The figure shows three views and two pictorial views of one solid part (mm, origin at its lowest corner). Answer the questions. A direction names the side the tool comes from. Coordinates: 2 decimals unless noted, no trailing zeros. Write each loop counter-clockwise with the first axis right and the second up, starting at its lowest first coordinate (ties: lowest second). Pieces come first, ordered by that corner, then holes. Notation, with made-up numbers: M 13.25,56 L 22.25,56 A9 ccw 22.25,63 Z; hole C 81,56 d6. An arc over 180 degrees is marked long. Use a Markdown table: item, result. Add a question column.
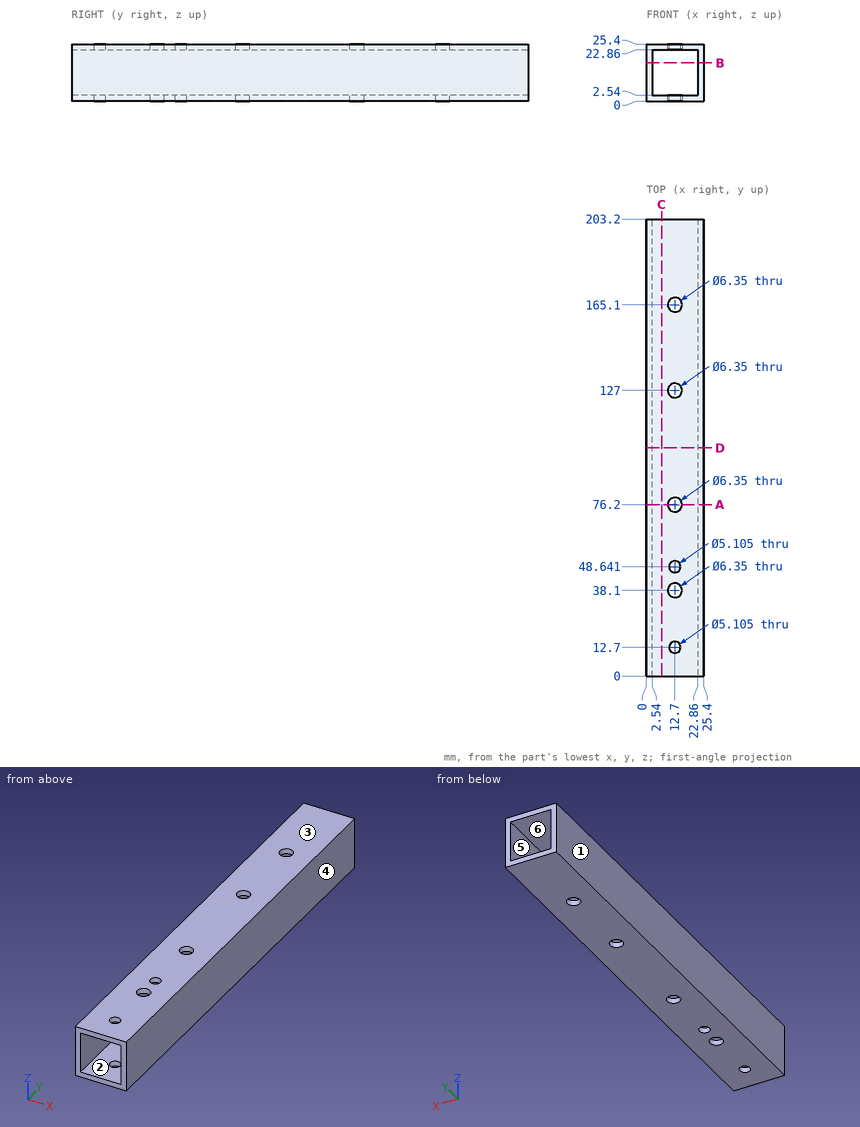
Item 1: Find section D-D on y = 101.5. Give the vertices of the cut face in (x, z), then the cut area to 3 significant figures.
Item 2: For the marked faces 1 and 2, determine the directions among +Z, -Z, +X, -X, +Y, -Y from which every point of the face is accessible in a straight line to the end or side of a thin tool.
Item 3: Consider probe 1 along Z at (x, y) = (17, 145); probe 2 along X at (y, z) = (165.1, 1.25) (1 decimal). Determine where each line is inside the solid, lowest interval first.
Item 4: Find section A-A on y = 76.2. Give the vertices of the cut face in (x, z) (1 decimal).
Item 5: Determine the mould class of the marked faces 3, 4, 5 and 6 for opening direction Z: pulls with the +Z half, pulls with the -Z half, needs draft (parallel to the pull), parting line crosses it, or undercut.
Item 6: Find section B-B on z = 17. Give the vertices of the cut face in (x, y), then the cut area to 3 significant figures.
Item 7: Find section C-C on x = 6.75. Give the vertices of the cut face in (y, z), then the cut area to 3 significant figures.
Geometry says:
| question | item | result |
|---|---|---|
| 1 | outline | M 0,0 L 25.4,0 L 25.4,25.4 L 0,25.4 Z; hole M 2.54,2.54 L 22.86,2.54 L 22.86,22.86 L 2.54,22.86 Z |
| 1 | area | 232 mm2 |
| 2 | face 1 | +Z, -Z, -X, +Y, -Y |
| 2 | face 2 | +Y, -Y |
| 3 | probe 1 | z = 0 to 2.54, 22.86 to 25.4 |
| 3 | probe 2 | x = 0 to 9.5, 15.9 to 25.4 |
| 4 | outline | M 0,0 L 9.5,0 L 9.5,2.5 L 2.5,2.5 L 2.5,22.9 L 9.5,22.9 L 9.5,25.4 L 0,25.4 Z; M 15.9,0 L 25.4,0 L 25.4,25.4 L 15.9,25.4 L 15.9,22.9 L 22.9,22.9 L 22.9,2.5 L 15.9,2.5 Z |
| 5 | face 3 | pulls with the +Z half |
| 5 | face 4 | needs draft |
| 5 | face 5 | undercut |
| 5 | face 6 | undercut |
| 6 | outline | M 0,0 L 2.54,0 L 2.54,203.2 L 0,203.2 Z; M 22.86,0 L 25.4,0 L 25.4,203.2 L 22.86,203.2 Z |
| 6 | area | 1,030 mm2 |
| 7 | outline | M 0,0 L 203.2,0 L 203.2,2.54 L 0,2.54 Z; M 0,22.86 L 203.2,22.86 L 203.2,25.4 L 0,25.4 Z |
| 7 | area | 1,030 mm2 |
